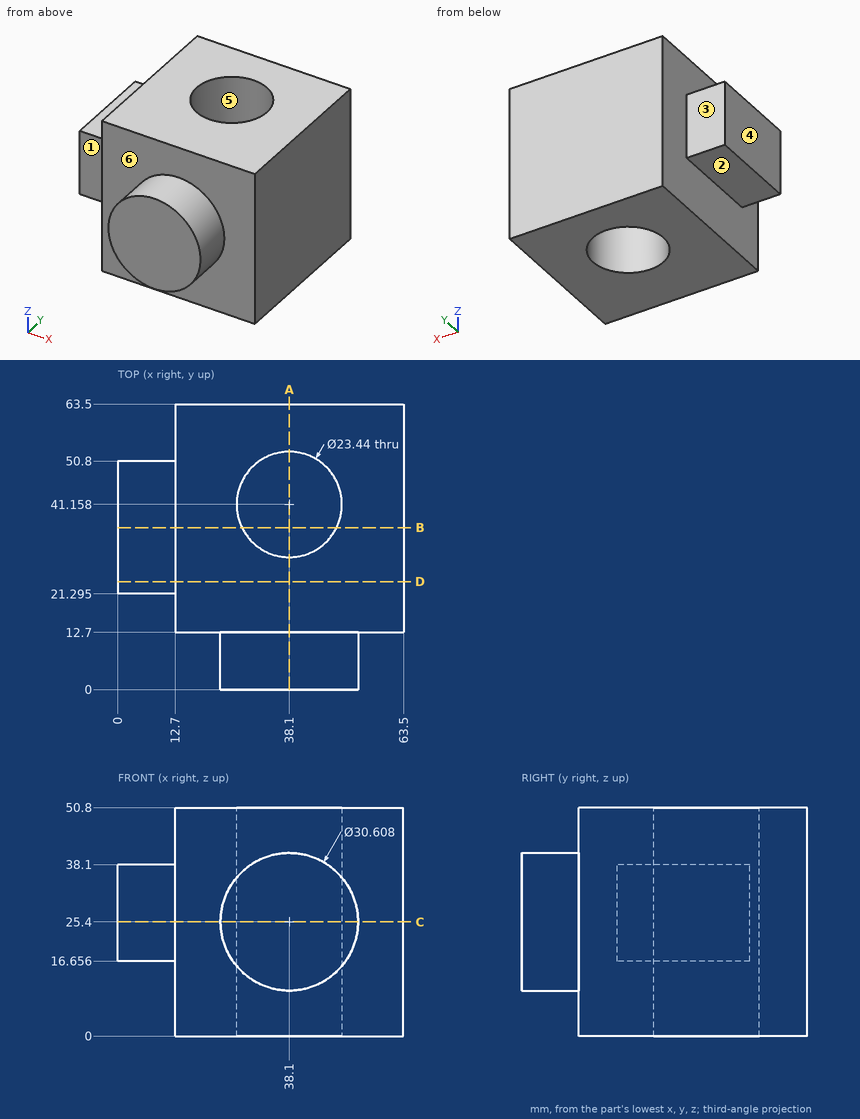
The drawing under review shows one solid part. Ordinate dimensions are in mm from its lowest x, y, z. A direction names the side the tool comes from. Round coordinates to 2 decimals unless told otherwise and drop trailing zeros. Write each loop counter-clockwise with the first axis right and the second up, starting at its lowest first coordinate (ties: lowest second). Pieces come first, ordered by that corner, then holes. Notation, with made-up numbers: (-17.75, -37.75) - (12.25, -37.75) arc R30 cw to (12.25, -1.75) - close; hole circle Ø7 at (84, 32.5). An arc over 180 degrees is marked (long way). Use a Markdown table: item, result. Add a question column.
1. We need section A-A (x = 38.1). State the section outline as (y, z) points, then the cut area to 3 significant figures.
2. Clearance check with flat-ended pins moving along their axes: pin 1 (6 mm diameter, centred on x = 15, z = 30.5, fed in from -Y); pin 2 (14 mm diameter, centred on x = 7, y = 42.5, fed in from -Z); pin 3 (4 mm diameter, centred on x = 3.5, z = 31.5, fed in from +Y); pin 4 (3 mm diameter, centred on y = 18.5, z = 27.5, fed in from -X). State where each tip first meets the part, or that it passes through.
3. We need section B-B (y = 36). State the section outline as (x, z) points, then the cut area to 3 significant figures.
4. We need section D-D (y = 24). State the section outline as (x, z) points, then the cut area to 3 significant figures.
5. For the marked faces 1, 2 and 3, list the 3-axis set-ups (+Z, -Z, +X, -X, +Y, -Y) from which the entire face can be reached by the end or side of a thin tool; tool diameter is ignored.
6. Wall thickness on probe 1 along Y at (x, z) = (38.1, 10); probe 2 along Y at (x, z) = (38.1, 16); probe 3 along X at (y, z) = (41, 26.5): over which ranges is each line inside the solid? List them lowest first.
7. We need section C-C (z = 25.4). State the section outline as (x, y) points (1 decimal), then the cut area to 3 significant figures.
8. Mouldability with a two-part tool opening along X and no side actions: class the marked faces 4, 5 and 6 as +X half, -X half, draft (parallel to the pull), parting line (faces both ways), or undercut.
Output:
| question | item | result |
|---|---|---|
| 1 | outline | (0, 10.1) - (12.7, 10.1) - (12.7, 0) - (29.44, 0) - (29.44, 50.8) - (12.7, 50.8) - (12.7, 40.7) - (0, 40.7) - close; (52.88, 0) - (63.5, 0) - (63.5, 50.8) - (52.88, 50.8) - close |
| 1 | area | 1,780 mm2 |
| 2 | pin 1 | stops at y = 12.7 |
| 2 | pin 2 | stops at z = 0 |
| 2 | pin 3 | stops at y = 50.8 |
| 2 | pin 4 | stops at x = 12.7 |
| 3 | outline | (0, 16.66) - (12.7, 16.66) - (12.7, 0) - (27.58, 0) - (27.58, 50.8) - (12.7, 50.8) - (12.7, 38.1) - (0, 38.1) - close; (48.62, 0) - (63.5, 0) - (63.5, 50.8) - (48.62, 50.8) - close |
| 3 | area | 1,780 mm2 |
| 4 | outline | (0, 16.66) - (12.7, 16.66) - (12.7, 0) - (63.5, 0) - (63.5, 50.8) - (12.7, 50.8) - (12.7, 38.1) - (0, 38.1) - close |
| 4 | area | 2,850 mm2 |
| 5 | face 1 | +Z, -Z, -X, -Y |
| 5 | face 2 | -Z, -X, +Y, -Y |
| 5 | face 3 | +Z, -Z, -X, +Y |
| 6 | probe 1 | y = 12.7 to 29.44, 52.88 to 63.5 |
| 6 | probe 2 | y = 0 to 29.44, 52.88 to 63.5 |
| 6 | probe 3 | x = 0 to 26.38, 49.82 to 63.5 |
| 7 | outline | (0, 21.3) - (12.7, 21.3) - (12.7, 12.7) - (22.8, 12.7) - (22.8, 0) - (53.4, 0) - (53.4, 12.7) - (63.5, 12.7) - (63.5, 63.5) - (12.7, 63.5) - (12.7, 50.8) - (0, 50.8) - close; hole circle Ø23.4 at (38.1, 41.2) |
| 7 | area | 2,910 mm2 |
| 8 | face 4 | -X half |
| 8 | face 5 | undercut |
| 8 | face 6 | draft |
